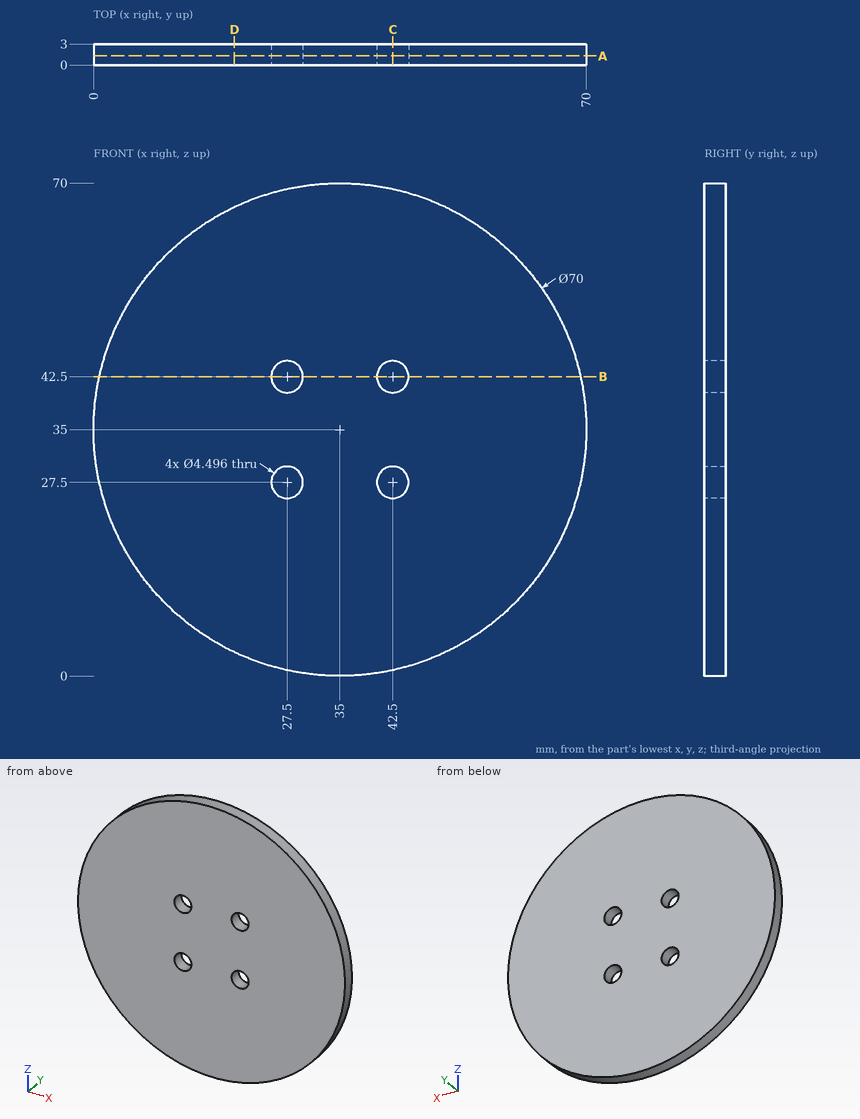
Answer from the drawing. Dimensions are ordinates in mm from the lowest x, y and z of the part. Give positions to 0.01 mm unless a question says otherwise; leave off trailing zeros. Loops run counter-clockwise (first coordinate to the right, second up) from the corner with the lowest first, then second, coordinate; pieces in that order, holes last. Notation, with made-up numbers: (-24.5, -1) -> (32.5, -1) arc R6 ccw to (32.5, 6) -> close; hole circle Ø6 at (13.25, 85). An arc over 180 degrees is marked (long way). Use a Markdown table: item, result.
Q1. Find the intervals of material crossed by line 1 along Z through (x, y) = (27, 1.8); line 2 along Z through (x, y) = (27.5, 0.85), in increasing order.
Solved:
| item | result |
|---|---|
| line 1 | z = 0.93 to 25.31, 29.69 to 40.31, 44.69 to 69.07 |
| line 2 | z = 0.81 to 25.25, 29.75 to 40.25, 44.75 to 69.19 |
Q2. Section C-C, the plane x = 42.5 is taken. Determine the outline of the cut face in (y, z).
Solved:
| item | result |
|---|---|
| outline | (0, 0.81) -> (3, 0.81) -> (3, 25.25) -> (0, 25.25) -> close; (0, 29.75) -> (3, 29.75) -> (3, 40.25) -> (0, 40.25) -> close; (0, 44.75) -> (3, 44.75) -> (3, 69.19) -> (0, 69.19) -> close |
Q3. Section D-D, the plane x = 20 is taken. Determine the outline of the cut face in (y, z), then the cut area to 3 significant figures.
Solved:
| item | result |
|---|---|
| outline | (0, 3.38) -> (3, 3.38) -> (3, 66.62) -> (0, 66.62) -> close |
| area | 190 mm^2 |
Q4. Section B-B, the plane z = 42.5 is taken. Determine the outline of the cut face in (x, y).
Solved:
| item | result |
|---|---|
| outline | (0.81, 0) -> (25.25, 0) -> (25.25, 3) -> (0.81, 3) -> close; (29.75, 0) -> (40.25, 0) -> (40.25, 3) -> (29.75, 3) -> close; (44.75, 0) -> (69.19, 0) -> (69.19, 3) -> (44.75, 3) -> close |
Q5. Section A-A, the plane y = 1.3 is taken. Determine the outline of the cut face in (x, z), then the cut area to 4 significant figures.
Solved:
| item | result |
|---|---|
| outline | circle Ø70 at (35, 35); hole circle Ø4.5 at (27.5, 27.5); hole circle Ø4.5 at (27.5, 42.5); hole circle Ø4.5 at (42.5, 27.5); hole circle Ø4.5 at (42.5, 42.5) |
| area | 3,785 mm^2 |
Q6. Each of these flat-tipped pins is pushed along its axis until it touches: pin 1 (2.5 mm diameter, centred on x = 42.5, z = 42.5, fed in from +Y); pin 2 (5 mm diameter, centred on x = 27.5, z = 42.5, fed in from +Y); pin 3 (1.5 mm diameter, centred on y = 0.5, z = 45, fed in from -X). Where does it stop, or does it pass through?
Solved:
| item | result |
|---|---|
| pin 1 | passes through |
| pin 2 | stops at y = 3 |
| pin 3 | stops at x = 1.24 |
